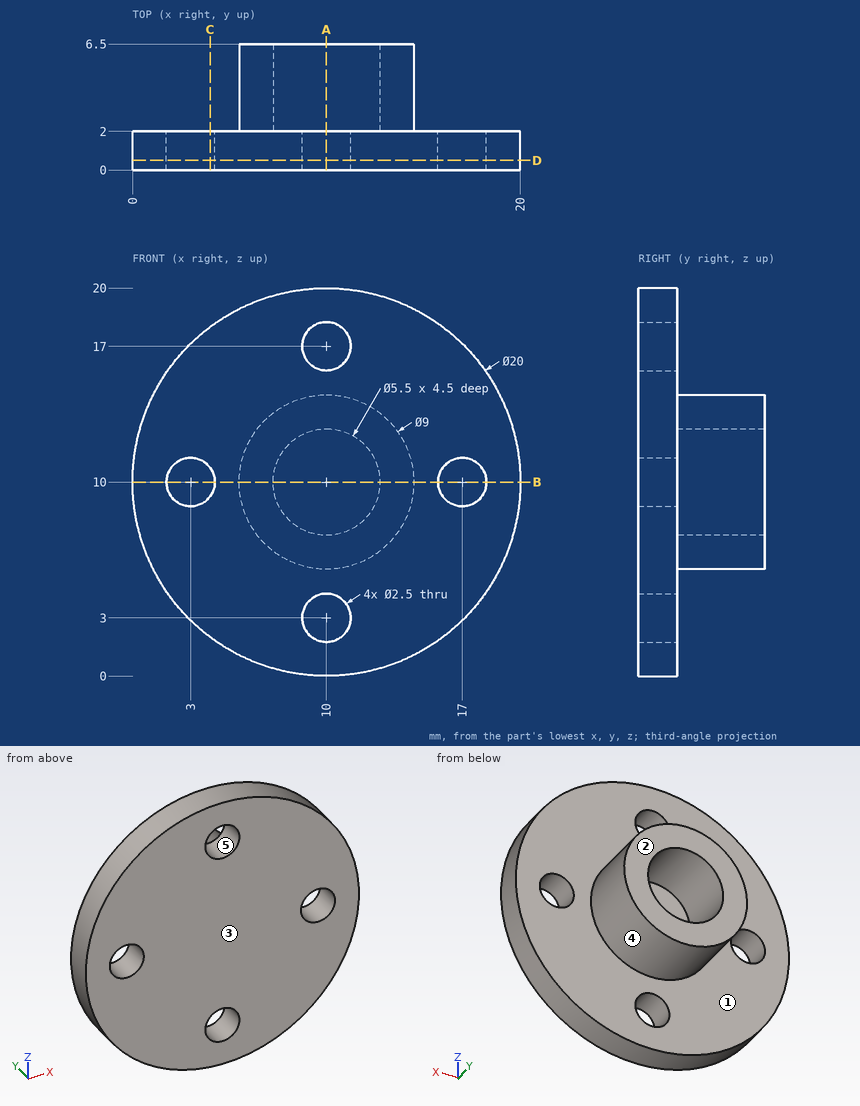
Study the drawing (mm; zero at the part's minimum x, y, z) and answer. A direction names the side the tool comes from. Give positions to 0.01 mm unless a question says otherwise; leave off trailing zeros. Loops run counter-clockwise (first coordinate to the right, second up) from the corner with the lowest first, then second, coordinate; pieces in that order, holes last. Notation, with made-up numbers: M -34,-22 L -7,-22 A19 cw -7,11 Z; hole C 3,10 d7. An arc over 180 degrees is marked long. Use CSV: the item, a comma, the result in double quotes.
1) Find section D-D on y = 0.5. Write down the section's boundary in (x, z).
Answer:
outline,"C 10,10 d20; hole C 3,10 d2.5; hole C 10,3 d2.5; hole C 10,17 d2.5; hole C 17,10 d2.5"
2) Find section B-B on z = 10. Write down the section's boundary in (x, y), plus the area to 4 significant figures.
Answer:
outline,"M 0,0 L 1.75,0 L 1.75,2 L 0,2 Z; M 4.25,0 L 15.75,0 L 15.75,2 L 14.5,2 L 14.5,6.5 L 12.75,6.5 L 12.75,2 L 7.25,2 L 7.25,6.5 L 5.5,6.5 L 5.5,2 L 4.25,2 Z; M 18.25,0 L 20,0 L 20,2 L 18.25,2 Z"
area,"45.75 mm^2"
3) Consider L1, parallel to X at y = 4.3, z = 10; L2, parallel to Z at x = 17, y = 0.5; L3, parallel to Y at x = 4.75, z = 8. Determine where each line is inside the solid, lowest interval first.
Answer:
L1,"5.5 to 7.25, 12.75 to 14.5"
L2,"2.86 to 8.75, 11.25 to 17.14"
L3,"0 to 2"
4) Given P1, Ø3, axis at x = 10, z = 3, coming from the +Y side; P2, Ø1.5, axis at y = 2.5, z = 15.5, coming from the +X side, each flat-ended and moving along its own axis, determine where each tip first touches the part or whether it passes through.
Answer:
P1,"y = 2"
P2,"x = 18.69"
5) Find section A-A on x = 10. Write down the section's boundary in (y, z).
Answer:
outline,"M 0,0 L 2,0 L 2,1.75 L 0,1.75 Z; M 0,4.25 L 2,4.25 L 2,5.5 L 6.5,5.5 L 6.5,7.25 L 2,7.25 L 2,12.75 L 6.5,12.75 L 6.5,14.5 L 2,14.5 L 2,15.75 L 0,15.75 Z; M 0,18.25 L 2,18.25 L 2,20 L 0,20 Z"
6) Which of the six approach directions +Z, -Z, +X, -X, +Y, -Y give full straight-line access (tool end or side, diameter ignored) to the marked faces 1 and 2?
Answer:
face 1,"+Y"
face 2,"+Z, -Z, +X, -X, +Y"
7) Find section C-C on x = 4. Write down the section's boundary in (y, z).
Answer:
outline,"M 0,2 L 2,2 L 2,9.25 L 0,9.25 Z; M 0,10.75 L 2,10.75 L 2,18 L 0,18 Z"
8) Determine the mould class of the marked faces 3, 4 and 5 for opening direction X: released by +X, released by -X, zero draft, split by the parting line, or undercut.
Answer:
face 3,"zero draft"
face 4,"split by the parting line"
face 5,"undercut"
